Study the drawing (mm; zero at the part's minimum x, y, z) and answer. A direction names the side the tool comes from. Give positions to 0.01 mm unless a question says otherwise; leave off trailing zeros. Loops run counter-clockwise (first coordinate to the right, second up) from the corner with the lowest first, then second, coordinate; pieces in that order, holes last. Notation, with made-up numbers: (-5, 48) - (15, 48) arc R4 cw to (15, 54) - close; hole circle Ø4 at (-2.75, 32.5). An arc over 180 degrees is marked (long way). Write item = value, one per line. Start each with the question number.
1) The part is cut by section D-D on x = 2.75. Write down the section's boundary in (y, z), plus the area to 3 significant figures.
2) Which of the six approach directions +Z, -Z, +X, -X, +Y, -Y give full straight-line access (tool end or side, diameter ignored) to the marked faces 5, 6, 7, 8 and 9?
3) A flat-ended cylindrical pin translates along its axis: P1, Ø1.5, axis at x = 6, z = 15.5, coming from the -Y side. Find the tip coordinate at first contact, or state that the pin passes through.
4) The part is cut by section A-A on z = 8.5. Write down the section's boundary in (x, y), plus the area to 3 significant figures.
5) The part is cut by section C-C on y = 11.5. Write down the section's boundary in (x, z), plus the area to 3 significant figures.
6) Consider probe 1 along Y at (x, z) = (16.75, 11); probe 2 along Z at (x, y) = (12, 23); probe 3 along Y at (x, z) = (10, 9.75). Determine where each line is inside the solid, lowest interval first.
7) The mould has two halves that part along Z. Classify the marked faces 1, 2, 3 and 4: +Z half, -Z half, draft (parallel to the pull), parting line (faces both ways), or undercut.
8) The part is cut by section B-B on x = 9.25. Write down the section's boundary in (y, z), plus the area to 3 significant figures.
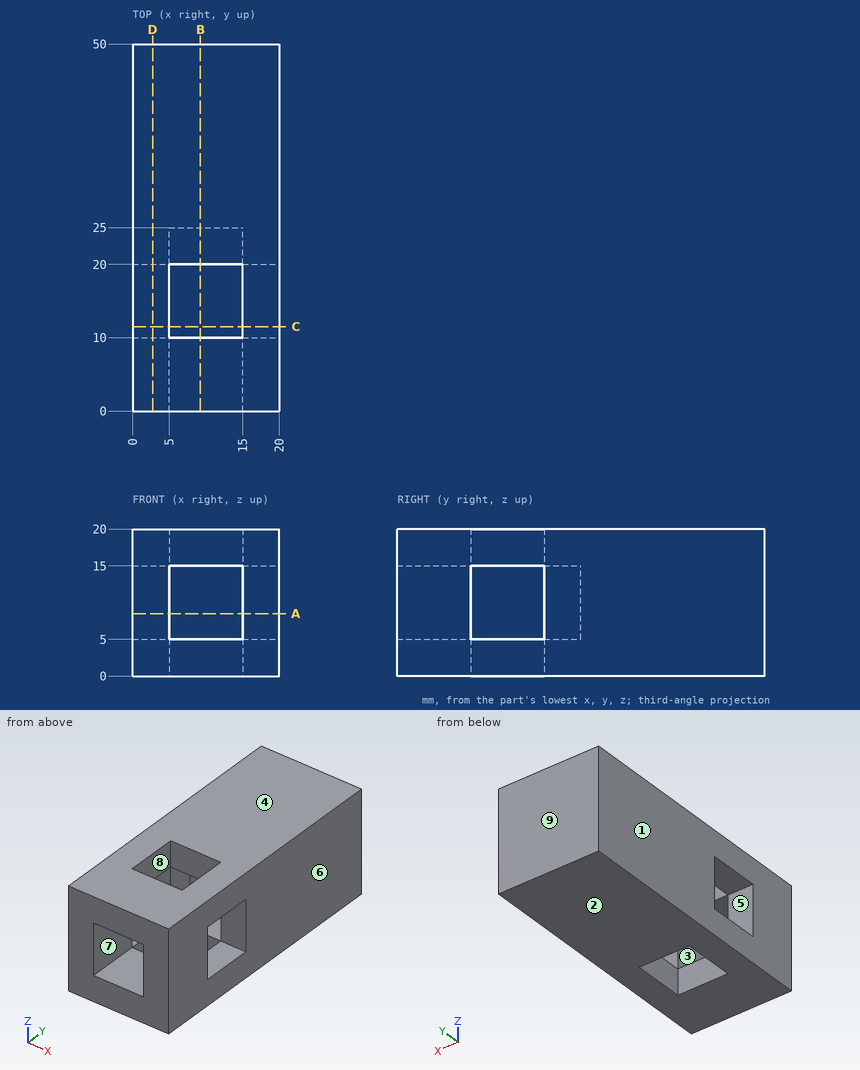
Answer below:
q1.outline = (0, 0) - (50, 0) - (50, 20) - (0, 20) - close; hole (10, 5) - (20, 5) - (20, 15) - (10, 15) - close
q1.area = 900 mm2
q2.face_5 = +X, -X
q2.face_6 = +Z, -Z, +X, +Y, -Y
q2.face_7 = -Y
q2.face_8 = +Z, -Z
q2.face_9 = +Z, -Z, +X, -X, +Y
q3.P1 = 0
q4.outline = (0, 0) - (5, 0) - (5, 10) - (0, 10) - close; (0, 20) - (5, 20) - (5, 25) - (15, 25) - (15, 20) - (20, 20) - (20, 50) - (0, 50) - close; (15, 0) - (20, 0) - (20, 10) - (15, 10) - close
q4.area = 650 mm2
q5.outline = (0, 0) - (5, 0) - (5, 5) - (0, 5) - close; (0, 15) - (5, 15) - (5, 20) - (0, 20) - close; (15, 0) - (20, 0) - (20, 5) - (15, 5) - close; (15, 15) - (20, 15) - (20, 20) - (15, 20) - close
q5.area = 100 mm2
q6.probe_1 = 0 to 10, 20 to 50
q6.probe_2 = 0 to 5, 15 to 20
q6.probe_3 = 25 to 50
q7.face_1 = draft
q7.face_2 = -Z half
q7.face_3 = undercut
q7.face_4 = +Z half
q8.outline = (0, 0) - (10, 0) - (10, 5) - (0, 5) - close; (0, 15) - (10, 15) - (10, 20) - (0, 20) - close; (20, 0) - (50, 0) - (50, 20) - (20, 20) - (20, 15) - (25, 15) - (25, 5) - (20, 5) - close
q8.area = 650 mm2
